Verification items for the finished model (mm, model axes). A direction names the side the tool comes from. Coordinates: 2 decimals unless noted, no trailing zeros. Order: outer loops, then holes, each group sorted by start corner. A loop starts at its lowest first (then second) coordinate and runs counter-clockwise, first axis right, second up. Notation, with made-up numbers: M 24,-25 L 62,-25 A18 cw 62,1 Z; hole C 87,-26 d9. An arc over 180 degrees is marked long. Answer as a JSON object with one key per item and string values. Group by question number.
(1) Material ranges on line 1 (Z direction, x = 3.75, y = -1.25) (3 decimals); line 2 (Y direction, x = -2, z = -18); line 3 (X direction, y = 0.25, z = -2), recorded low to high.
(2) Access from +Z, -Z, +X, -X, +Y, -Y to the whole of each face (thin tool, end or side, straight path). Record for faces 1 (the face through (0, 0, -35)), 2 (the face through (-0.83, -3.72, -17.26)).
(3) Cross-section at C-C (z = -21). Enter the section's corners in (x, y), plus the area to 3 significant figures.
(4) Gauge pin test, flat ends, axial feed: pin 1 Ø6 at (x, z) = (3, -28.5) entering from +Y; pin 2 Ø4 at (y, z) = (-4.5, -20) entering from -X; pin 3 Ø4 at (x, y) = (-4, 0.5) entering from -Z. Record the tip position at first contact, or that the pin passes through.
(5) Cross-section at D-D (z = 0.5). Enter the section's corners in (x, y).
from build123d import *

# Parameters (mm, degrees)
SKETCH1_R           = 3.81
BASE_EXTRUDE_DEPTH  = 35
SKETCH2_R           = 6.35
BOSS_EXTRUDE1_DEPTH = 3.175
FILLET1_R           = 1.5875


with BuildPart() as part:
    # Sketch1 → Base-Extrude (new body)
    with BuildSketch(Plane.XY):
        Circle(SKETCH1_R)
    extrude(amount=-BASE_EXTRUDE_DEPTH)

    # Sketch2 → Boss-Extrude1 (add)
    with BuildSketch(Plane.XY):
        Circle(SKETCH2_R)
    extrude(amount=BOSS_EXTRUDE1_DEPTH)

    # Fillet1
    fillet1_edges = [part.edges().sort_by_distance(p)[0] for p in [
        (-6.35, 0, 3.175),
    ]]
    fillet(fillet1_edges, radius=FILLET1_R)


solid = part.part
Taken from the geometry:
{
 "1": {"line 1": "z = 0 to 3.175", "line 2": "y = -3.24 to 3.24", "line 3": "x = -3.8 to 3.8"},
 "2": {"face 1": "-Z, +X, -X, +Y, -Y", "face 2": "-Z"},
 "3": {"outline": "C 0,0 d7.62", "area": "45.6 mm²"},
 "4": {"pin 1": "stops at y = 3.81", "pin 2": "stops at x = -2.88", "pin 3": "stops at z = -35"},
 "5": {"outline": "C 0,0 d12.7"}
}
